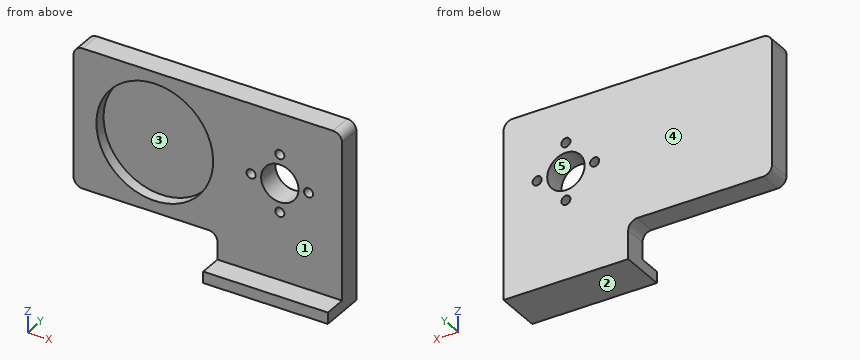
from build123d import *

# Parameters (mm, degrees)
SKETCH1_W           = 74.754
SKETCH1_H           = 38.862
SKETCH1_R           = 5.207
SKETCH1_R_2         = 16.256
SKETCH1_W_2         = 34.7
SKETCH1_H_2         = 10.541
BOSS_EXTRUDE1_DEPTH = 6.35
BOSS_EXTRUDE2_START = -3.175
SKETCH2_R           = 16.256
BOSS_EXTRUDE2_DEPTH = 3.175
SKETCH3_W           = 34.7
SKETCH3_H           = 3.175
BOSS_EXTRUDE3_DEPTH = 12.7
FILLET1_R           = 2.54
SKETCH4_R           = 1.27
CUT_EXTRUDE1_DEPTH  = 65.944794531


with BuildPart() as part:
    # Sketch1 → Boss-Extrude1 (new body)
    # profile 1 of 2: a face of its own
    with BuildSketch(Plane(origin=(0, 0, 0), x_dir=(1, 0, 0), z_dir=(0, 1, 0))):
        with Locations((-4.886569512, -28.216948841)):
            Rectangle(SKETCH1_W, SKETCH1_H)
        with Locations(Location((15.140430488, -28.216948841, 0), (0, 0, 270))):
            Circle(SKETCH1_R, mode=Mode.SUBTRACT)
        with Locations(Location((-19.657569512, -28.216948841, 0), (0, 0, 270))):
            Circle(SKETCH1_R_2, mode=Mode.SUBTRACT)
    # profile 2 of 2: a face of its own
    with BuildSketch(Plane(origin=(0, 0, 0), x_dir=(1, 0, 0), z_dir=(0, 1, 0))):
        with Locations((15.140430488, -3.515448841)):
            Rectangle(SKETCH1_W_2, SKETCH1_H_2)
    extrude(amount=BOSS_EXTRUDE1_DEPTH)

    # Sketch2 → Boss-Extrude2 (add)
    with BuildSketch(Plane(origin=(0, 6.35, 0), x_dir=(1, 0, 0), z_dir=(0, 1, 0)).offset(BOSS_EXTRUDE2_START)):
        with Locations(Location((-19.657569512, -28.216948841, 0), (0, 0, 270))):
            Circle(SKETCH2_R)
    extrude(amount=BOSS_EXTRUDE2_DEPTH)

    # Sketch3 → Boss-Extrude3 (add)
    with BuildSketch(Plane(origin=(0, 6.35, 0), x_dir=(1, 0, 0), z_dir=(0, 1, 0))):
        with Locations((15.140430488, 0.167551159)):
            Rectangle(SKETCH3_W, SKETCH3_H)
    extrude(amount=-BOSS_EXTRUDE3_DEPTH)

    # Fillet1
    fillet1_edges = [part.edges().sort_by_distance(p)[0] for p in [
        (32.490430488, 3.175, 47.647948841),
        (-42.263569512, 3.175, 47.647948841),
        (-42.263569512, 3.175, 8.785948841),
        (-2.209569512, 3.175, 8.785948841),
    ]]
    fillet(fillet1_edges, radius=FILLET1_R)

    # Sketch4 → Cut-Extrude1 (cut, through all)
    with BuildSketch(Plane(origin=(0, 6.35, 0), x_dir=(1, 0, 0), z_dir=(0, 1, 0))):
        with Locations(Location((15.140430488, -20.215948841, 0), (0, 0, 270))):
            Circle(SKETCH4_R)
        with Locations(Location((23.141430488, -28.216948841, 0), (0, 0, 270))):
            Circle(SKETCH4_R)
        with Locations(Location((15.140430488, -36.217948841, 0), (0, 0, 270))):
            Circle(SKETCH4_R)
        with Locations(Location((7.139430488, -28.216948841, 0), (0, 0, 270))):
            Circle(SKETCH4_R)
    extrude(amount=-CUT_EXTRUDE1_DEPTH, mode=Mode.SUBTRACT)


solid = part.part
Here's how the part is built. I have some questions about the finished solid (model axes, mm). Face numbers are marked on the shaded views. A direction names the side the tool comes from. Round coordinates to 2 decimals unless told otherwise and drop trailing zeros. Write each loop counter-clockwise with the first axis right and the second up, starting at its lowest first coordinate (ties: lowest second). Pieces come first, ordered by that corner, then holes.
1. For the marked faces 1, 2 and 3, which set-ups out of +Z, -Z, +X, -X, +Y, -Y let a thin tool reach every point of the face, with its end or its side?
2. Suppose I cut it at C-C (y = 1.75). List the corners of the cut face in (x, z) for me, and give its area (3 significant figures).
3. Suppose I cut it at B-B (x = 18.5). List the corners of the cut face in (y, z) for me, and give its area (3 significant figures).
4. Will these pins go through, and if not, where does the flat tip stop? pin 1 Ø14 at (x, z) = (-22.5, 15.5) entering from -Y; pin 2 Ø6.5 at (y, z) = (3, 3) entering from -X; pin 3 Ø3 at (x, y) = (9.5, -3) entering from +Z.
5. I need wall thicknesses on L1, parallel to Z at x = -19.5, y = 2; L2, parallel to X at y = 1, z = 28.5; L3, parallel to X at y = 1.25, z = 27.5. Which ranges of each line are inside material? Lowest first, please.
6. If we mould it in two halves opening along X, with no side actions, what happens to the marked faces 4 and 5? For each: released by +X, released by -X, zero draft, split by the parting line, or undercut.
7. Suppose I cut it at A-A (z = 31). List the corners of the cut face in (x, y) for me (3 decimals), and give its area (3 significant figures).
8. Suppose I cut it at D-D (x = 26.5). List the corners of the cut face in (y, z) for me, and give its area (3 significant figures).
Answer sheet:
1. face 1: +Z, +X, -X, -Y
1. face 2: -Z, +X, -X, +Y, -Y
1. face 3: -Y
2. outline: (-42.26, 11.33) arc R2.54 ccw to (-39.72, 8.79) - (-4.75, 8.79) arc R2.54 cw to (-2.21, 6.25) - (-2.21, -1.76) - (32.49, -1.76) - (32.49, 45.11) arc R2.54 ccw to (29.95, 47.65) - (-39.72, 47.65) arc R2.54 ccw to (-42.26, 45.11) - close; hole circle Ø32.51 at (-19.66, 28.22); hole circle Ø2.54 at (7.14, 28.22); hole circle Ø10.41 at (15.14, 28.22); hole circle Ø2.54 at (15.14, 20.22); hole circle Ø2.54 at (15.14, 36.22); hole circle Ø2.54 at (23.14, 28.22)
2. area: 2,330 mm2
3. outline: (-6.35, -1.76) - (6.35, -1.76) - (6.35, 24.24) - (0, 24.24) - (0, 1.42) - (-6.35, 1.42) - close; (0, 32.2) - (6.35, 32.2) - (6.35, 47.65) - (0, 47.65) - close
3. area: 283 mm2
4. pin 1: stops at y = 0
4. pin 2: stops at x = -2.21
4. pin 3: stops at z = 1.42
5. L1: z = 8.79 to 11.96, 44.47 to 47.65
5. L2: x = -42.26 to -35.91, -3.4 to 5.9, 8.38 to 9.94, 20.34 to 21.9, 24.38 to 32.49
5. L3: x = -42.26 to -35.9, -3.42 to 6.09, 8.19 to 9.98, 20.3 to 22.09, 24.19 to 32.49
6. face 4: zero draft
6. face 5: undercut
7. outline: (-42.264, 0) - (-35.674, 0) - (-35.674, 3.175) - (-3.642, 3.175) - (-3.642, 0) - (10.74, 0) - (10.74, 6.35) - (-42.264, 6.35) - close; (19.541, 0) - (32.49, 0) - (32.49, 6.35) - (19.541, 6.35) - close
7. area: 317 mm2
8. outline: (-6.35, -1.76) - (6.35, -1.76) - (6.35, 47.65) - (0, 47.65) - (0, 1.42) - (-6.35, 1.42) - close
8. area: 334 mm2
